```python
from build123d import *

# Parameters (mm, degrees)
SKETCH1_W           = 47
SKETCH1_H           = 42.2
BOSS_EXTRUDE1_DEPTH = 4.5
FILLET1_R           = 20


with BuildPart() as part:
    # Sketch1 → Boss-Extrude1 (new body)
    with BuildSketch(Plane(origin=(0, 0, 0), x_dir=(1, 0, 0), z_dir=(0, 1, 0))):
        Polygon((0, 0), (-69.282032303, -40), (-34.641016151, -100), (69.282032303, -40), align=None)
        Polygon((-19.457626094, -24.098403011), (4.042373906, -64.801596989), (-32.503898133, -85.901596989), (-56.003898133, -45.198403011), (-55.051270189, -44.648403011), (-57.076270189, -41.141000126), (-22.435254038, -21.141000126), (-20.410254038, -24.648403011), align=None, mode=Mode.SUBTRACT)
        Polygon((4.042373906, -64.801596989), (-19.457626094, -24.098403011), (-56.003898133, -45.198403011), (-32.503898133, -85.901596989), align=None)
        Polygon((103.923048454, 20), (0, 80), (-69.282032303, 80), (-69.282032303, -40), (0, 0), (69.282032303, -40), align=None)
        Polygon((-11.141016151, 28.9), (-58.141016151, 28.9), (-58.141016151, 71.1), (-11.141016151, 71.1), (-11.141016151, 70), (-7.091016151, 70), (-7.091016151, 30), (-11.141016151, 30), align=None, mode=Mode.SUBTRACT)
        Polygon((30.598642245, -4.801596989), (54.098642245, 35.901596989), (90.644914285, 14.801596989), (67.144914285, -25.901596989), (66.192286341, -25.351596989), (64.167286341, -28.858999874), (29.526270189, -8.858999874), (31.551270189, -5.351596989), align=None, mode=Mode.SUBTRACT)
        with Locations((-34.641016151, 50)):
            Rectangle(SKETCH1_W, SKETCH1_H)
        Polygon((54.098642245, 35.901596989), (30.598642245, -4.801596989), (67.144914285, -25.901596989), (90.644914285, 14.801596989), align=None)
    extrude(amount=BOSS_EXTRUDE1_DEPTH)

    # Fillet1
    fillet1_edges = [part.edges().sort_by_distance(p)[0] for p in [
        (-69.282032303, 2.25, -80),
        (0, 2.25, -80),
        (103.923048454, 2.25, -20),
        (69.282032303, 2.25, 40),
        (-34.641016151, 2.25, 100),
        (-69.282032303, 2.25, 40),
    ]]
    fillet(fillet1_edges, radius=FILLET1_R)


solid = part.part
```
For this review, take the finished solid that the model builds, in its own axes (mm). A direction names the side the tool comes from. Coordinates: 2 decimals unless noted, no trailing zeros. Order: outer loops, then holes, each group sorted by start corner. A loop starts at its lowest first (then second) coordinate and runs counter-clockwise, first axis right, second up. Notation, with made-up numbers: (72.5, 2) - (87.5, 2) arc R20 ccw to (87.5, 24) - close; hole circle Ø5 at (86, 84.25). An arc over 180 degrees is marked (long way). Answer as a JSON object with one key per item and string values. Group by question number.
1. We need section C-C on x = 59. State the section outline as (y, z) points, then the cut area to 3 significant figures.
2. For faces 4 (the flat face through (-7.091, 2, -50)), 5 (the cylindrical face through (-68.58, 2.28, 39.89)), list the 3-axis set-ups (+Z, -Z, +X, -X, +Y, -Y) from which the entire face can be reached by the end or side of a thin tool; tool diameter is ignored.
3. The part is to be moulded in two halves that separate along Z. For faces 1 (the flat face through (47.09, 2.22, 19)), 2 (the cylindrical face through (-0.11, 2.28, -79.3)), 3 (the flat face through (23.09, 2.22, 66.67)), say which applies: pulls with the +Z half, pulls with the -Z half, needs draft (parallel to the pull), parting line crosses it, or undercut.
4. Clearance check with flat-ended pins moving along their axes: P1, Ø1.5, axis at y = 2.5, z = -52.5, coming from the +X side; P2, Ø2, axis at x = -9, y = 1.5, coming from the +Z side; P3, Ø2, axis at y = 3, z = -57.5, coming from the +X side. State where each tip first meets the part, or that it passes through.
5. We need section D-D on x = 0. State the section outline as (y, z) points.
6. For probe 1 along X at (y, z) = (3.55, 27); probe 2 along Z at (x, y) = (41, 3.4); probe 3 along X at (y, z) = (2.45, -36), list the stretches that pass through material, from the lowest coordinate up.
7. We need section A-A on y = 3.5. State the section outline as (x, z) points, then the cut area to 3 significant figures.
8. We need section B-B on z = 12. State the section outline as (x, y) points, then the cut area to 3 significant figures.
Final values:
{
 "1": {"outline": "(0, -45.94) - (4.5, -45.94) - (4.5, 21.2) - (0, 21.2) - close; (0, 25.88) - (4.5, 25.88) - (4.5, 45.94) - (0, 45.94) - close", "area": "392 mm²"},
 "2": {"face 4": "+Y, -Y", "face 5": "+Z, -X, +Y, -Y"},
 "3": {"face 1": "undercut", "face 2": "pulls with the -Z half", "face 3": "pulls with the +Z half"},
 "4": {"P1": "x = 48.93", "P2": "z = 85.77", "P3": "x = 40.7"},
 "5": {"outline": "(0, -79.27) - (4.5, -79.27) - (4.5, 80) - (0, 80) - close"},
 "6": {"probe 1": "-69.28 to -32.58, -24.48 to 60.95, 65.24 to 76.79", "probe 2": "-56.33 to 10.81, 15.48 to 56.33", "probe 3": "-69.28 to -11.14, -7.09 to 76.21"},
 "7": {"outline": "(-69.28, -60) arc R20 ccw to (-49.28, -80) - (-5.36, -80) arc R20 ccw to (4.64, -77.32) - (86.6, -30) arc R20 ccw to (93.92, -2.68) - (71.96, 35.36) arc R20 ccw to (64.64, 42.68) - (-17.32, 90) arc R20 ccw to (-44.64, 82.68) - (-66.6, 44.64) arc R20 ccw to (-69.28, 34.64) - close; hole (-57.08, 41.14) - (-22.44, 21.14) - (-20.41, 24.65) - (-55.05, 44.65) - close; hole (-11.14, -70) - (-7.09, -70) - (-7.09, -30) - (-11.14, -30) - close; hole (29.53, 8.86) - (31.55, 5.35) - (66.19, 25.35) - (64.17, 28.86) - close", "area": "20,000 mm²"},
 "8": {"outline": "(-69.28, 0) - (34.97, 0) - (34.97, 4.5) - (-69.28, 4.5) - close; (43.07, 0) - (85.45, 0) - (85.45, 4.5) - (43.07, 4.5) - close", "area": "660 mm²"}
}
